For this review, take the finished solid that the model builds, in its own axes (mm). A direction names the side the tool comes from. Coordinates: 2 decimals unless noted, no trailing zeros. Order: outer loops, then holes, each group sorted by start corner. A loop starts at its lowest first (then second) coordinate and runs counter-clockwise, first axis right, second up. Notation, with made-up numbers: (44, 75) -> (98, 75) arc R18 cw to (98, 83) -> close; hole circle Ø9 at (58, 39.5). An arc over 180 degrees is marked (long way). Answer as a JSON object with one key per item and string values. Group by question number.
1) Wall thickness on L1, parallel to X at y = 0.7, z = 0; L2, parallel to Z at x = 58, y = 0.9; L3, parallel to Y at x = -13, z = 4.5: over which ranges is each line inside the solid? List them lowest first.
2) Add section A-A, the plane x = 0. Write out the cut boundary in (y, z).
3) Add section C-C, the plane x = -52. Write out the cut boundary in (y, z).
4) For pin 1 (3 mm diameter, centred on x = 20.5, y = 4, fed in from +Z); pin 2 (2 mm diameter, centred on y = 3.5, z = 1, fed in from -X); pin 3 (6 mm diameter, centred on x = -27, z = -4, fed in from +Y); pin 4 (1.5 mm diameter, centred on y = 7, z = 1, fed in from +X), all flat-tipped, find the tip position at first contact; note any pin that passes through.
5) Add section B-B, the plane y = 15.25. Write out the cut boundary in (x, z).
6) Draft analysis for pull direction Z (two halves, no side actions). For faces 3 (the cylindrical face through (63, 1, 0)), 4 (the flat face through (-1, 1, -5)), 5 (the cylindrical face through (-56.153, 0.986, 0.766)), state which applies: +Z half, -Z half, draft (parallel to the pull), parting line (faces both ways), or undercut.
7) Machinability: for faces 1 (the flat face through (1, 0, 0)), 2 (the cylindrical face through (-0.54, 9.4, 2.44)), which of the approach directions +Z, -Z, +X, -X, +Y, -Y give a long, thin tool a straight path to every point of the face, cutting with its end or side? Answer none if there is none.
from build123d import *

# Parameters (mm, degrees)
SKETCH1_R           = 2
BOSS_EXTRUDE1_DEPTH = 2
SKETCH2_R           = 2.5
BOSS_EXTRUDE2_DEPTH = 15


with BuildPart() as part:
    # Sketch1 → Boss-Extrude1 (new body)
    with BuildSketch(Plane(origin=(0, 0, 0), x_dir=(1, 0, 0), z_dir=(0, 1, 0))):
        with BuildLine():
            Line((-58, 5), (58, 5))
            ThreePointArc((58, 5), (63, 0), (58, -5))
            Line((58, -5), (-58, -5))
            ThreePointArc((-58, -5), (-63, 0), (-58, 5))
        make_face()
        with Locations((-58, 0)):
            Circle(SKETCH1_R, mode=Mode.SUBTRACT)
        with Locations((58, 0)):
            Circle(SKETCH1_R, mode=Mode.SUBTRACT)
    extrude(amount=BOSS_EXTRUDE1_DEPTH)

    # Sketch2 → Boss-Extrude2 (add)
    with BuildSketch(Plane(origin=(0, 2, 0), x_dir=(1, 0, 0), z_dir=(0, 1, 0))):
        Circle(SKETCH2_R)
    extrude(amount=BOSS_EXTRUDE2_DEPTH)


solid = part.part
Output values:
{
 "1": {"L1": "x = -63 to -60, -56 to 56, 60 to 63", "L2": "z = -5 to -2, 2 to 5", "L3": "y = 0 to 2"},
 "2": {"outline": "(0, -5) -> (2, -5) -> (2, -2.5) -> (17, -2.5) -> (17, 2.5) -> (2, 2.5) -> (2, 5) -> (0, 5) -> close"},
 "3": {"outline": "(0, -5) -> (2, -5) -> (2, 5) -> (0, 5) -> close"},
 "4": {"pin 1": "passes through", "pin 2": "stops at x = -2.5", "pin 3": "stops at y = 2", "pin 4": "stops at x = 2.49"},
 "5": {"outline": "circle Ø5 at (0, 0)"},
 "6": {"face 3": "parting line", "face 4": "-Z half", "face 5": "undercut"},
 "7": {"face 1": "+Z, -Z, +X, -X, -Y", "face 2": "+Y"}
}
